Build history of the part. All positions in model axes, mm. A direction names the side the tool comes from. Round coordinates to 2 decimals unless told otherwise and drop trailing zeros. Order: outer loops, then holes, each group sorted by start corner. A loop starts at its lowest first (then second) coordinate and runs counter-clockwise, first axis right, second up. Notation, with made-up numbers: (-5.5, 33.5) -> (3.5, 33.5) arc R23 cw to (3.5, 70.5) -> close; hole circle Ø8 at (-30.5, 61.25). An arc over 180 degrees is marked (long way). Answer as a JSON object with one key per item and string values.
from build123d import *

# Parameters (mm, degrees)
SKETCH1_R           = 17.375
BOSS_EXTRUDE1_DEPTH = 17.7
SKETCH7_R           = 13.545
CUT_EXTRUDE4_DEPTH  = 5
SKETCH10_R          = 3.485
BOSS_EXTRUDE3_DEPTH = 1
SKETCH11_R          = 1.65
CUT_EXTRUDE5_DEPTH  = 13.7


with BuildPart() as part:
    # Sketch1 → Boss-Extrude1 (new body)
    with BuildSketch(Plane(origin=(0, 0, 0), x_dir=(1, 0, 0), z_dir=(0, 1, 0))):
        Circle(SKETCH1_R)
    extrude(amount=BOSS_EXTRUDE1_DEPTH)

    # Sketch7 → Cut-Extrude4 (cut)
    with BuildSketch(Plane.XZ):
        Circle(SKETCH7_R)
    extrude(amount=-CUT_EXTRUDE4_DEPTH, mode=Mode.SUBTRACT)

    # Sketch10 → Boss-Extrude3 (add)
    with BuildSketch(Plane.XZ.offset(-5)):
        Circle(SKETCH10_R)
    extrude(amount=BOSS_EXTRUDE3_DEPTH)

    # Sketch11 → Cut-Extrude5 (cut)
    with BuildSketch(Plane.XZ.offset(-4)):
        Circle(SKETCH11_R)
    extrude(amount=-CUT_EXTRUDE5_DEPTH, mode=Mode.SUBTRACT)


solid = part.part
1) Cut at B-B, the plane x = 0. Give the cut face in (y, z) (3 decimals).
Checked values:
{"outline": "(0, -17.375) -> (17.7, -17.375) -> (17.7, -1.65) -> (4, -1.65) -> (4, -3.485) -> (5, -3.485) -> (5, -13.545) -> (0, -13.545) -> close; (0, 13.545) -> (5, 13.545) -> (5, 3.485) -> (4, 3.485) -> (4, 1.65) -> (17.7, 1.65) -> (17.7, 17.375) -> (0, 17.375) -> close"}
2) Cut at D-D, the plane z = -6.5. Give the cut face in (x, y).
Checked values:
{"outline": "(-16.11, 0) -> (-11.88, 0) -> (-11.88, 5) -> (11.88, 5) -> (11.88, 0) -> (16.11, 0) -> (16.11, 17.7) -> (-16.11, 17.7) -> close"}
3) Cut at C-C, the plane y = 14.75. Give the cut face in (x, z) (3 decimals), plus the area to 3 significant figures.
Checked values:
{"outline": "circle Ø34.75 at (0, 0); hole circle Ø3.3 at (0, 0)", "area": "940 mm²"}
4) Which spindle directions (+Z, -Z, +X, -X, +Y, -Y) get a long thin tool onto all of the face, cutting with end or side? Do faces 4 (the face through (-5, 0, 13)), 5 (the face through (1.61, 4.51, -3.09)). Say none if no direction does.
Checked values:
{"face 4": "+Z, -Z, +X, -X, -Y", "face 5": "-Y"}
5) Cut at A-A, the plane z = 0. Give the cut face in (x, y) (3 decimals).
Checked values:
{"outline": "(-17.375, 0) -> (-13.545, 0) -> (-13.545, 5) -> (-3.485, 5) -> (-3.485, 4) -> (-1.65, 4) -> (-1.65, 17.7) -> (-17.375, 17.7) -> close; (1.65, 4) -> (3.485, 4) -> (3.485, 5) -> (13.545, 5) -> (13.545, 0) -> (17.375, 0) -> (17.375, 17.7) -> (1.65, 17.7) -> close"}
6) Pull direction Z, two halves, no side cores. Call faces 1 (the face through (4, 17.7, 0)), 2 (the face through (-1.216, 10.754, 1.115)), 3 (the face through (9.34, 8.73, -14.65)): pulls with the +Z half, pulls with the -Z half, needs draft (parallel to the pull), parting line crosses it, or undercut.
Checked values:
{"face 1": "needs draft", "face 2": "undercut", "face 3": "parting line crosses it"}
7) Flat gauge pins, fed straight in: pin 1 Ø5 at (x, y) = (7, 12.5) entering from -Z; pin 2 Ø4 at (x, z) = (0, 0) entering from -Y; pin 3 Ø4 at (y, z) = (12, -7) entering from -X. Where does each tip first touch, or does it go through?
Checked values:
{"pin 1": "stops at z = -16.78", "pin 2": "stops at y = 4", "pin 3": "stops at x = -16.64"}
8) Probe L1, parallel to Z at x = 0, y = 1.5 (3 decimals); L2, parallel to Y at x = -5, z = -3.5; L3, parallel to Z at x = 0, y = 8.75 (3 decimals). List the from-to ranges inside material, lowest first. Write a range as from..to.
Checked values:
{"L1": "z = -17.375..-13.545, 13.545..17.375", "L2": "y = 5..17.7", "L3": "z = -17.375..-1.65, 1.65..17.375"}
